CAD build for the part. Positions are in the model's coordinates, mm. A direction names the side the tool comes from. Give positions to 0.01 mm unless a question says otherwise; leave off trailing zeros. Loops run counter-clockwise (first coordinate to the right, second up) from the corner with the lowest first, then second, coordinate; pieces in that order, holes last. Notation, with made-up numbers: (79, 72) -> (92, 72) arc R23 cw to (92, 102) -> close; hole circle Ø4 at (36.25, 57). An arc over 180 degrees is marked (long way). Write each question's results on one line, items separated by ' | '. Start each with the question number.
```python
from build123d import *

# Parameters (mm, degrees)
F1_DEPTH = 6.35
F2_R     = 3.175
F3_DEPTH = 1.27
F5_DEPTH = 25.4


with BuildPart() as f1:
    # F0 (on Front) → F1 (new body, symmetric)
    with BuildSketch(Plane.XZ):
        Polygon((-25.4, 25.4), (0, 0), (0, 25.4), align=None)
    extrude(amount=F1_DEPTH, both=True)

    # F2 (on face) → F3 (cut)
    with BuildSketch(Plane(origin=(0, 0, 0), x_dir=(0.7071067812, 0, -0.7071067812), z_dir=(-0.7071067812, 0, -0.7071067812))):
        with Locations((-13.97, 0)):
            Circle(F2_R)
        with Locations((-6.35, 0)):
            Circle(F2_R)
    extrude(amount=-F3_DEPTH, mode=Mode.SUBTRACT)

    # F4 (on face) → F5 (cut)
    with BuildSketch(Plane.YZ):
        with BuildLine():
            ThreePointArc((6.1483610621, 25.4), (10.9401596307, 30.0624684299), (12.7, 36.5125))
            ThreePointArc((12.7, 36.5125), (-6.4500315701, 47.4526596307), (-6.1483610621, 25.4))
            Line((-6.1483610621, 25.4), (6.1483610621, 25.4))
        make_face()
        with BuildLine():
            Line((6.1483610621, 25.4), (-6.1483610621, 25.4))
            ThreePointArc((-6.1483610621, 25.4), (0, 23.8125), (6.1483610621, 25.4))
        make_face()
    extrude(amount=-F5_DEPTH, mode=Mode.SUBTRACT)


solid = f1.part
```
Q1. Saw through at C-C, the plane y = -3.5. List the corners of the cut face in (x, z).
Q2. Saw through at B-B, the plane z = 16.5. List the corners of the cut face in (x, y), then the cut area to 3 significant figures.
Q3. Wall check: L1, parallel to Y at x = -10.75, z = 11.5; L2, parallel to Z at x = -7.5, y = -0.25; L3, parallel to Z at x = -13.75, y = -3.5. Give the ranges that are in metal, low to high.
Q4. Saw through at D-D, the plane x = -20. List the corners of the cut face in (y, z), then the cut area to 3 significant figures.
Q5. Saw through at A-A, the plane x = -16. List the corners of the cut face in (y, z).
Q6. Drop flat-ended pins along their axis: pin 1 (1 mm diameter, centred on y = -4, z = 22, fed in from -X); pin 2 (1.5 mm diameter, centred on x = -22, y = 2, fed in from -Z); pin 3 (3 mm diameter, centred on x = -3, y = -4.5, fed in from -Z). Give the stop position or say it passes through.
Q7. Which spindle directions (+Z, -Z, +X, -X, +Y, -Y) get a long thin tool onto all of the face, cutting with end or side? Do faces 1 (the face through (-12.522, -0.09, 23.813)), 2 (the face through (-9.012, -0.044, 10.808)). Say none if no direction does.
Q8. Mould opens along Z. For faces 3 (the face through (-13, 0, 13)), 4 (the face through (0, 0, 13)), 5 (the face through (-3.624, -0.044, 5.42)) say: pulls with the +Z half, pulls with the -Z half, needs draft (parallel to the pull), parting line crosses it, or undercut.
Answer block:
1) outline: (-24.3, 24.3) -> (0, 0) -> (0, 24.3) -> close
2) outline: (-16.5, -6.35) -> (0, -6.35) -> (0, 6.35) -> (-16.5, 6.35) -> close | area: 210 mm2
3) L1: y = -6.35 to -2.64, 2.64 to 6.35 | L2: z = 7.5 to 7.78, 9.3 to 23.81 | L3: z = 13.75 to 24.3
4) outline: (-6.35, 20) -> (6.35, 20) -> (6.35, 25.4) -> (6.15, 25.4) arc R12.7 cw to (-6.15, 25.4) -> (-6.35, 25.4) -> close | area: 55.4 mm2
5) outline: (-6.35, 16) -> (6.35, 16) -> (6.35, 25.4) -> (6.15, 25.4) arc R12.7 cw to (-6.15, 25.4) -> (-6.35, 25.4) -> close
6) pin 1: stops at x = -22.5 | pin 2: stops at z = 21.25 | pin 3: stops at z = 1.5
7) face 1: +Z, +X, -X | face 2: none
8) face 3: pulls with the -Z half | face 4: needs draft | face 5: undercut
